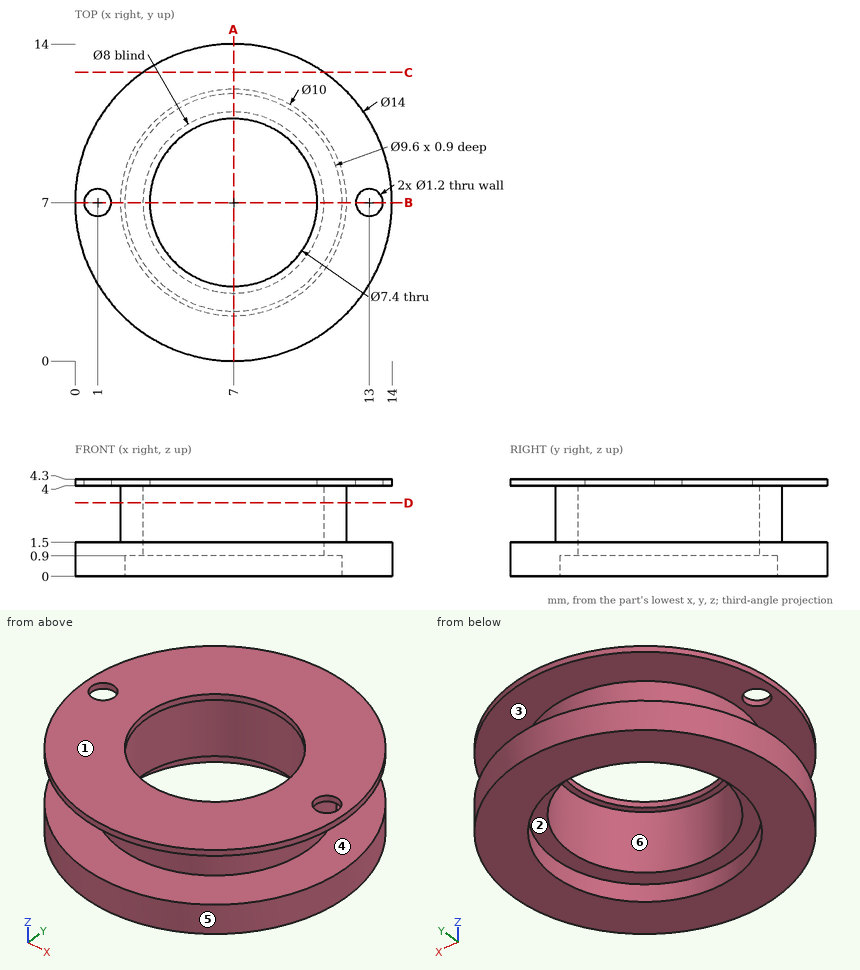
Study the drawing (mm; zero at the part's minimum x, y, z) and answer. A direction names the side the tool comes from. Give positions to 0.01 mm unless a question says otherwise; leave off trailing zeros. Loops run counter-clockwise (first coordinate to the right, second up) from the corner with the lowest first, then second, coordinate; pieces in that order, holes last. Notation, with made-up numbers: M 9,-38.5 L 44,-38.5 A30 cw 44,-0.5 Z; hole C -17.75,57 d6. An arc over 180 degrees is marked long. One line per item, written item: value. Start each with the question number.
1. Determine the mould class of the marked faces 4, 5 and 6 for opening direction X: released by +X, released by -X, zero draft, split by the parting line, or undercut.
2. Find section C-C (y = 12.75). Give the vertices of the cut face in (x, z), and give its area (3 significant figures).
3. Which of the six approach directions +Z, -Z, +X, -X, +Y, -Y give full straight-line access (tool end or side, diameter ignored) to the marked faces 1, 2 and 3?
4. Find the intervals of material crossed by probe 1 along Y at (x, z) = (7, 0.7); probe 2 along Y at (x, z) = (7, 3.1); probe 3 along Z at (x, y) = (1.5, 3), in increasing order.
5. Find section B-B (y = 7). State how many separate pieces and enclosed holes the cut face has, and give its area (3 significant figures).
6. Find section A-A (x = 7). Give the vertices of the cut face in (y, z).
7. Each of these flat-tipped pins is pushed along its axis until it touches: P1, Ø1.5, axis at y = 11, z = 3, coming from the -X side; P2, Ø1.1, axis at x = 13, y = 7, coming from the +Z side; P3, Ø5, axis at x = 5.5, y = 6.5, coming from the -Z side. Where does it stop, or does it pass through?
8. Find section D-D (z = 3.25). Give the vertices of the cut face in (x, y), and give its area (3 significant figures).
Reported:
1. face 4: zero draft
1. face 5: split by the parting line
1. face 6: undercut
2. outline: M 3.01,0 L 10.99,0 L 10.99,1.5 L 3.01,1.5 Z; M 3.01,4 L 10.99,4 L 10.99,4.3 L 3.01,4.3 Z
2. area: 14.4 mm²
3. face 1: +Z, +X, -X, +Y, -Y
3. face 2: -Z
3. face 3: none
4. probe 1: y = 0 to 2.2, 11.8 to 14
4. probe 2: y = 2 to 3, 11 to 12
4. probe 3: z = 0 to 1.5, 4 to 4.3
5. separate pieces: 4
5. enclosed holes: 0
5. area: 13.8 mm²
6. outline: M 0,0 L 2.2,0 L 2.2,0.9 L 3,0.9 L 3,4 L 3.3,4 L 3.3,4.3 L 0,4.3 L 0,4 L 2,4 L 2,1.5 L 0,1.5 Z; M 10.7,4 L 11,4 L 11,0.9 L 11.8,0.9 L 11.8,0 L 14,0 L 14,1.5 L 12,1.5 L 12,4 L 14,4 L 14,4.3 L 10.7,4.3 Z
7. P1: stops at x = 3.2
7. P2: stops at z = 1.5
7. P3: stops at z = 0.9
8. outline: C 7,7 d10; hole C 7,7 d8
8. area: 28.3 mm²
